Design review of the part shown in the three views and the two pictorial views. Dimensions are in mm from the part's minimum x, y and z. Coordinates: 2 decimals unless noted, no trailing zeros. Loops run counter-clockwise (first coordinate to the right, second up) from the corner with the lowest first, then second, coordinate; pieces in that order, holes last. Notation, with made-up numbers: (28, 36) -> (37, 36) arc R25 cw to (37, 69) -> close; hole circle Ø10 at (-9, 59.25). An arc over 180 degrees is marked (long way). One line per item, written item: value. Start each with the question number.
1. Add section B-B on x = 365. Write out the cut boundary in (y, z) (3 decimals), plus the area to 3 significant figures.
2. For probe 1 along X at (y, z) = (122, 4.25); probe 2 along Y at (x, z) = (148, 2.8) (3 decimals); probe 3 along X at (y, z) = (99.5, 4.2) (3 decimals), list the stretches that pass through material, from the lowest coordinate up.
3. Insertion check: pin 1 (3 mm diameter, centred on x = 116, z = 2, fed in from +Y) (3 decimals); pin 2 (1.7 mm diameter, centred on y = 43.5, z = 2.5, fed in from -X) (3 decimals); pin 3 (1.7 mm diameter, centred on x = 61, z = 2, fed in from -Y) (3 decimals). Each pin has a flat end and moves straight along its axis. Give the tip position at first contact, or say it passes through.
4. Add section A-A on y = 85.5. Write out the cut boundary in (x, z) (3 decimals), plus the area to 3 significant figures.
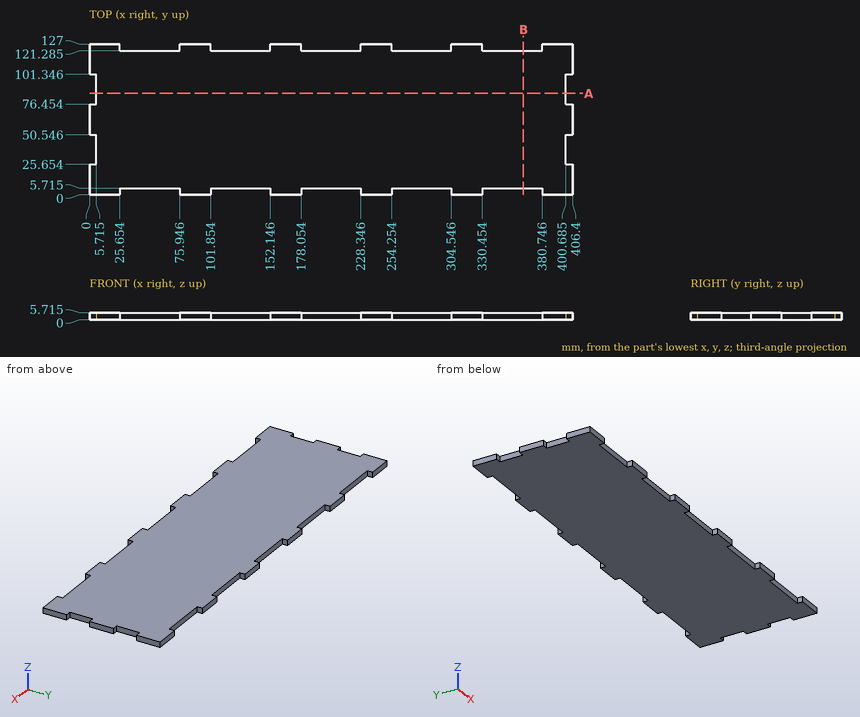
Worked answers:
1. outline: (5.715, 0) -> (121.285, 0) -> (121.285, 5.715) -> (5.715, 5.715) -> close
1. area: 660 mm²
2. probe 1: x = 0 to 25.65, 75.95 to 101.85, 152.15 to 178.05, 228.35 to 254.25, 304.55 to 330.45, 380.75 to 406.4
2. probe 2: y = 5.715 to 121.285
2. probe 3: x = 5.715 to 400.685
3. pin 1: stops at y = 121.285
3. pin 2: stops at x = 5.715
3. pin 3: stops at y = 5.715
4. outline: (5.715, 0) -> (400.685, 0) -> (400.685, 5.715) -> (5.715, 5.715) -> close
4. area: 2,260 mm²
